```python
from build123d import *

# Parameters (mm, degrees)
F1_DEPTH = 30
F2_R     = 1.5
F3_DEPTH = 4.001
F4_SIZE  = 15
F5_DEPTH = 2


with BuildPart() as f1:
    # F0 (on Top) → F1 (new body, symmetric)
    with BuildSketch(Plane.XY):
        with BuildLine():
            ThreePointArc((-5.25, 0), (-4.130678, 3.24037), (-1.25, 5.09902))
            Line((-1.25, 5.09902), (-1.25, 40))
            Line((-1.25, 40), (-5.25, 40))
            Line((-5.25, 40), (-5.25, 0))
        make_face()
        with BuildLine():
            ThreePointArc((5.25, 0), (3.24037, 4.130678), (-1.25, 5.09902))
            ThreePointArc((-1.25, 5.09902), (-4.130678, 3.24037), (-5.25, 0))
            ThreePointArc((-5.25, 0), (0, -5.25), (5.25, 0))
        make_face()
        with BuildLine():
            ThreePointArc((-1.25, 0), (0, 1.25), (1.25, 0))
            ThreePointArc((1.25, 0), (0, -1.25), (-1.25, 0))
        make_face(mode=Mode.SUBTRACT)
    extrude(amount=F1_DEPTH, both=True)

    # F2 (on face) → F3 (cut, through all)
    with BuildSketch(Plane.YZ.offset(-1.25)):
        with Locations((22, 8)):
            Circle(F2_R)
        with Locations((29, 0)):
            Circle(F2_R)
        with Locations((22, -8)):
            Circle(F2_R)
    extrude(amount=-F3_DEPTH, mode=Mode.SUBTRACT)

    # F4
    f4_edges = [f1.edges().sort_by_distance(p)[0] for p in [
        (-3.25, 40, 30),
        (-3.25, 40, -30),
    ]]
    chamfer(f4_edges, length=F4_SIZE)

    # F2 (on face) → F5 (cut)
    with BuildSketch(Plane.YZ.offset(-1.25)):
        Polygon((23.587713, 10.75), (20.412287, 10.75), (18.824574, 8), (20.412287, 5.25), (23.587713, 5.25), (25.175426, 8), align=None)
        with Locations((22, 8)):
            Circle(F2_R, mode=Mode.SUBTRACT)
        Polygon((30.587713, 2.75), (27.412287, 2.75), (25.824574, 0), (27.412287, -2.75), (30.587713, -2.75), (32.175426, 0), align=None)
        with Locations((29, 0)):
            Circle(F2_R, mode=Mode.SUBTRACT)
        Polygon((23.587713, -5.25), (20.412287, -5.25), (18.824574, -8), (20.412287, -10.75), (23.587713, -10.75), (25.175426, -8), align=None)
        with Locations((22, -8)):
            Circle(F2_R, mode=Mode.SUBTRACT)
    extrude(amount=-F5_DEPTH, mode=Mode.SUBTRACT)


solid = f1.part
```
Model file for the job. Use its own axes, mm. A direction names the side the tool comes from. Give positions to 0.01 mm unless a question says otherwise; leave off trailing zeros. Write each loop counter-clockwise with the first axis right and the second up, starting at its lowest first coordinate (ties: lowest second). Pieces come first, ordered by that corner, then holes. Notation, with made-up numbers: (23, -12.75) -> (78, -12.75) arc R21 cw to (78, 12.25) -> close; hole circle Ø1 at (38, 24). An arc over 180 degrees is marked (long way). Use CSV: the item, a comma, the result in double quotes. Start each with the question number.
1) Cut at D-D on y = 16.5. List the corners of the cut face in (x, z).
2) Two-plate mould, pull along Z, no slides. Class faces 3 (the flat face through (-2.24, 24.39, -6.64)), 4 (the flat face through (-3, 33, -22)), 5 (the cylindrical face through (-4.24, 27.5, 0.07)), 6 (the flat face through (-2, 7, 30)): released by +Z, released by -Z, zero draft, split by the parting line, or undercut.
3) Drill centre lines: L1, parallel to Z at x = -4.2, y = 22; L2, parallel to Z at x = -2.75, y = 20.5; L3, parallel to Y at x = 0, z = 11. Where is each one in solid material? Low to high.
4) Cut at B-B on y = 29. List the corners of the cut face in (x, z), plus the area to 3 significant figures.
5) Tool access for faces 1 (the cylindrical face through (-4.2, 20.8, -8.9)), 2 (the flat face through (-2, 22, -5.25)): list every direction of +Z, -Z, +X, -X, +Y, -Y with a clear straight run to the whole face (end or side of a thin tool).
6) Pin check, flat tips, straight feed: P1, Ø17.5, axis at y = 23.5, z = -11.5, coming from the +X side; P2, Ø1, axis at x = 0.5, y = 14.5, coming from the +Z side; P3, Ø2, axis at x = -2.5, y = 29, coming from the +Z side; P4, Ø4, axis at y = 4.5, z = 21, coming from the +X side. Stop position of each tip, or through.
7) Cut at A-A on x = 0. List the corners of the cut face in (y, z).
8) Cut at C-C on z = -20.5. List the corners of the cut face in (x, y), plus the area to 3 significant figures.
Final values:
1,outline,"(-5.25, -30) -> (-1.25, -30) -> (-1.25, 30) -> (-5.25, 30) -> close"
2,face 3,"undercut"
2,face 4,"released by -Z"
2,face 5,"undercut"
2,face 6,"released by +Z"
3,L1,"z = -30 to -9.5, -6.5 to 6.5, 9.5 to 30"
3,L2,"z = -30 to -10.75, -5.25 to 5.25, 10.75 to 30"
3,L3,"y = -5.25 to -1.25, 1.25 to 5.25"
4,outline,"(-5.25, -26) -> (-1.25, -26) -> (-1.25, -2.75) -> (-3.25, -2.75) -> (-3.25, -1.5) -> (-5.25, -1.5) -> close; (-5.25, 1.5) -> (-3.25, 1.5) -> (-3.25, 2.75) -> (-1.25, 2.75) -> (-1.25, 26) -> (-5.25, 26) -> close"
4,area,"191 mm2"
5,face 1,"+X, -X"
5,face 2,"+X"
6,P1,"stops at x = -1.25"
6,P2,"passes through"
6,P3,"stops at z = 27"
6,P4,"stops at x = 4.62"
7,outline,"(-5.25, -30) -> (-1.25, -30) -> (-1.25, 30) -> (-5.25, 30) -> close; (1.25, -30) -> (5.25, -30) -> (5.25, 30) -> (1.25, 30) -> close"
8,outline,"(-5.25, 0) arc R5.25 ccw (long way) to (-1.25, 5.1) -> (-1.25, 34.5) -> (-5.25, 34.5) -> close; hole circle Ø2.5 at (0, 0)"
8,area,"205 mm2"
